from build123d import *

# Parameters (mm, degrees)
SKETCH_2_W            = 36.9
SKETCH_2_H            = 60.6
SKETCH_2_W_2          = 33.7
SKETCH_2_H_2          = 57.4
SKETCH_2_R            = 3.75
SKETCH_2_R_2          = 2.25
SKETCH_2_R_3          = 0.75
EXTRUDE_1_DEPTH       = 1.5
EXTRUDE_2_OUTLINE_R   = 2.154871705
EXTRUDE_2_DEPTH       = 3
EXTRUDE_2_DRAFT       = 28
EXTRUDE_2_2_OUTLINE_R = 2.154871705
EXTRUDE_2_2_DEPTH     = 3
EXTRUDE_2_2_DRAFT     = 28
EXTRUDE_2_3_DEPTH     = 3
EXTRUDE_2_3_DRAFT     = 28
EXTRUDE_2_4_OUTLINE_R = 2.154871705
EXTRUDE_2_4_DEPTH     = 3
EXTRUDE_2_4_DRAFT     = 28
EXTRUDE_START         = 1.5
SKETCH_2_11_W         = 36.9
SKETCH_2_11_H         = 60.6
SKETCH_2_11_W_2       = 33.7
SKETCH_2_11_H_2       = 57.4
EXTRUDE_3_DEPTH       = 4.5
SKETCH_3_W            = 1.6
SKETCH_3_H            = 5.7
SKETCH_3_H_2          = 5.5
EXTRUDE_4_DEPTH       = 4.3
SKETCH_5_W            = 0.8
SKETCH_5_H            = 5.5
SKETCH_5_H_2          = 5.7
EXTRUDE_5_DEPTH       = 1.5
CUT_EXTRUDE_START     = 1.5
SKETCH_2_12_R         = 0.75
CUT_EXTRUDE_1_DEPTH   = 3


# Read off the part's stored shape, not the designer's step: Бобышка-Вытянуть2
with BuildPart() as part:
    # Эскиз2 → Бобышка-Вытянуть1 (new body)
    # profile 1 of 14: a face of its own
    with BuildSketch(Plane(origin=(0, 0, 0), x_dir=(1, 0, 0), z_dir=(0, 1, 0))):
        with Locations((16.65, 28.5)):
            Rectangle(SKETCH_2_W, SKETCH_2_H)
        with Locations((16.65, 28.5)):
            Rectangle(SKETCH_2_W_2, SKETCH_2_H_2, mode=Mode.SUBTRACT)
    # profile 2 of 14: a face of its own
    with BuildSketch(Plane(origin=(0, 0, 0), x_dir=(1, 0, 0), z_dir=(0, 1, 0))):
        with BuildLine():
            Line((-0.2, 57.2), (-0.2, -0.2))
            Line((-0.2, -0.2), (33.5, -0.2))
            Line((33.5, -0.2), (33.5, 10.050490243))
            ThreePointArc((33.5, 10.050490243), (27, 12.6), (33.5, 15.149509757))
            Line((33.5, 15.149509757), (33.5, 57.2))
            Line((33.5, 57.2), (-0.2, 57.2))
        make_face()
        with Locations((5.1, 19.73)):
            Circle(SKETCH_2_R, mode=Mode.SUBTRACT)
        with Locations((5.1, 41.13)):
            Circle(SKETCH_2_R, mode=Mode.SUBTRACT)
        with Locations((23.55, 45)):
            Circle(SKETCH_2_R, mode=Mode.SUBTRACT)
    # profile 3 of 14: a face of its own
    with BuildSketch(Plane(origin=(0, 0, 0), x_dir=(1, 0, 0), z_dir=(0, 1, 0))):
        with Locations((23.55, 45)):
            Circle(SKETCH_2_R)
        with Locations((23.55, 45)):
            Circle(SKETCH_2_R_2, mode=Mode.SUBTRACT)
    # profile 4 of 14: a face of its own
    with BuildSketch(Plane(origin=(0, 0, 0), x_dir=(1, 0, 0), z_dir=(0, 1, 0))):
        with Locations((23.55, 45)):
            Circle(SKETCH_2_R_2)
        with Locations((23.55, 45)):
            Circle(SKETCH_2_R_3, mode=Mode.SUBTRACT)
    # profile 5 of 14: a face of its own
    with BuildSketch(Plane(origin=(0, 0, 0), x_dir=(1, 0, 0), z_dir=(0, 1, 0))):
        with Locations((23.55, 45)):
            Circle(SKETCH_2_R_3)
    # profile 6 of 14: a face of its own
    with BuildSketch(Plane(origin=(0, 0, 0), x_dir=(1, 0, 0), z_dir=(0, 1, 0))):
        with Locations((5.1, 41.13)):
            Circle(SKETCH_2_R)
        with Locations((5.1, 41.13)):
            Circle(SKETCH_2_R_2, mode=Mode.SUBTRACT)
    # profile 7 of 14: a face of its own
    with BuildSketch(Plane(origin=(0, 0, 0), x_dir=(1, 0, 0), z_dir=(0, 1, 0))):
        with Locations((5.1, 41.13)):
            Circle(SKETCH_2_R_2)
        with Locations((5.1, 41.13)):
            Circle(SKETCH_2_R_3, mode=Mode.SUBTRACT)
    # profile 8 of 14: a face of its own
    with BuildSketch(Plane(origin=(0, 0, 0), x_dir=(1, 0, 0), z_dir=(0, 1, 0))):
        with Locations((5.1, 41.13)):
            Circle(SKETCH_2_R_3)
    # profile 9 of 14: a face of its own
    with BuildSketch(Plane(origin=(0, 0, 0), x_dir=(1, 0, 0), z_dir=(0, 1, 0))):
        with Locations((5.1, 19.73)):
            Circle(SKETCH_2_R)
        with Locations((5.1, 19.73)):
            Circle(SKETCH_2_R_2, mode=Mode.SUBTRACT)
    # profile 10 of 14: a face of its own
    with BuildSketch(Plane(origin=(0, 0, 0), x_dir=(1, 0, 0), z_dir=(0, 1, 0))):
        with Locations((5.1, 19.73)):
            Circle(SKETCH_2_R_2)
        with Locations((5.1, 19.73)):
            Circle(SKETCH_2_R_3, mode=Mode.SUBTRACT)
    # profile 11 of 14: a face of its own
    with BuildSketch(Plane(origin=(0, 0, 0), x_dir=(1, 0, 0), z_dir=(0, 1, 0))):
        with Locations((5.1, 19.73)):
            Circle(SKETCH_2_R_3)
    # profile 12 of 14: a face of its own
    with BuildSketch(Plane(origin=(0, 0, 0), x_dir=(1, 0, 0), z_dir=(0, 1, 0))):
        with BuildLine():
            ThreePointArc((33.5, 15.149509757), (27, 12.6), (33.5, 10.050490243))
            Line((33.5, 10.050490243), (33.5, 15.149509757))
        make_face()
        with Locations((30.75, 12.6)):
            Circle(SKETCH_2_R_2, mode=Mode.SUBTRACT)
    # profile 13 of 14: a face of its own
    with BuildSketch(Plane(origin=(0, 0, 0), x_dir=(1, 0, 0), z_dir=(0, 1, 0))):
        with Locations((30.75, 12.6)):
            Circle(SKETCH_2_R_2)
        with Locations((30.75, 12.6)):
            Circle(SKETCH_2_R_3, mode=Mode.SUBTRACT)
    # profile 14 of 14: a face of its own
    with BuildSketch(Plane(origin=(0, 0, 0), x_dir=(1, 0, 0), z_dir=(0, 1, 0))):
        with Locations((30.75, 12.6)):
            Circle(SKETCH_2_R_3)
    extrude(amount=EXTRUDE_1_DEPTH)


with BuildPart() as extrude_2_tool:
    # Бобышка-Вытянуть2 outline → Бобышка-Вытянуть2 (with draft: the straight prism first)
    with BuildSketch(Plane(origin=(0, 4.5, 0), x_dir=(1, 0, 0), z_dir=(0, 1, 0))):
        with Locations((5.1, 41.13)):
            Circle(EXTRUDE_2_OUTLINE_R)
    extrude(amount=-EXTRUDE_2_DEPTH)
    # Бобышка-Вытянуть2: the draft: its side faces are tilted about the plane it starts from
    extrude_2_sides = [extrude_2_tool.faces().sort_by_distance(p)[0] for p in [
        (2.945128295, 3, -41.13),
    ]]
    draft(extrude_2_sides, Plane(origin=(0, 4.5, 0), x_dir=(1, 0, 0), z_dir=(0, 1, 0)), EXTRUDE_2_DRAFT)


with BuildPart() as part_1:
    add(part.part)

    # Бобышка-Вытянуть2: add extrude_2_tool
    add(extrude_2_tool.part)


with BuildPart() as extrude_2_2_tool:
    # Extrude 2 2 outline → Extrude 2 2 (with draft: the straight prism first)
    with BuildSketch(Plane(origin=(0, 4.5, 0), x_dir=(1, 0, 0), z_dir=(0, 1, 0))):
        with Locations((23.55, 45)):
            Circle(EXTRUDE_2_2_OUTLINE_R)
    extrude(amount=-EXTRUDE_2_2_DEPTH)
    # Extrude 2 2: the draft: its side faces are tilted about the plane it starts from
    extrude_2_2_sides = [extrude_2_2_tool.faces().sort_by_distance(p)[0] for p in [
        (21.395128295, 3, -45),
    ]]
    draft(extrude_2_2_sides, Plane(origin=(0, 4.5, 0), x_dir=(1, 0, 0), z_dir=(0, 1, 0)), EXTRUDE_2_2_DRAFT)


with BuildPart() as part_2:
    add(part_1.part)

    # Extrude 2 2: add extrude_2_2_tool
    add(extrude_2_2_tool.part)


with BuildPart() as extrude_2_3_tool:
    # Extrude 2 3 outline → Extrude 2 3 (with draft: the straight prism first)
    with BuildSketch(Plane(origin=(0, 4.5, 0), x_dir=(1, 0, 0), z_dir=(0, 1, 0))):
        with BuildLine():
            ThreePointArc((31.904871705, 14.419270021), (28.595128295, 12.6), (31.904871705, 10.780729979))
            Line((31.904871705, 10.780729979), (31.904871705, 14.419270021))
        make_face()
    extrude(amount=-EXTRUDE_2_3_DEPTH)
    # Extrude 2 3: the draft: its side faces are tilted about the plane it starts from
    extrude_2_3_sides = [extrude_2_3_tool.faces().sort_by_distance(p)[0] for p in [
        (28.595128295, 3, -12.6),
        (31.904871705, 3, -12.6),
    ]]
    draft(extrude_2_3_sides, Plane(origin=(0, 4.5, 0), x_dir=(1, 0, 0), z_dir=(0, 1, 0)), EXTRUDE_2_3_DRAFT)


with BuildPart() as part_3:
    add(part_2.part)

    # Extrude 2 3: add extrude_2_3_tool
    add(extrude_2_3_tool.part)


with BuildPart() as extrude_2_4_tool:
    # Extrude 2 4 outline → Extrude 2 4 (with draft: the straight prism first)
    with BuildSketch(Plane(origin=(0, 4.5, 0), x_dir=(1, 0, 0), z_dir=(0, 1, 0))):
        with Locations((5.1, 19.73)):
            Circle(EXTRUDE_2_4_OUTLINE_R)
    extrude(amount=-EXTRUDE_2_4_DEPTH)
    # Extrude 2 4: the draft: its side faces are tilted about the plane it starts from
    extrude_2_4_sides = [extrude_2_4_tool.faces().sort_by_distance(p)[0] for p in [
        (2.945128295, 3, -19.73),
    ]]
    draft(extrude_2_4_sides, Plane(origin=(0, 4.5, 0), x_dir=(1, 0, 0), z_dir=(0, 1, 0)), EXTRUDE_2_4_DRAFT)


with BuildPart() as part_4:
    add(part_3.part)

    # Extrude 2 4: add extrude_2_4_tool
    add(extrude_2_4_tool.part)

    # Эскиз2<11> → Бобышка-Вытянуть3 (add)
    with BuildSketch(Plane(origin=(0, 0, 0), x_dir=(1, 0, 0), z_dir=(0, 1, 0)).offset(EXTRUDE_START)):
        with Locations((16.65, 28.5)):
            Rectangle(SKETCH_2_11_W, SKETCH_2_11_H)
        with Locations((16.65, 28.5)):
            Rectangle(SKETCH_2_11_W_2, SKETCH_2_11_H_2, mode=Mode.SUBTRACT)
    extrude(amount=EXTRUDE_3_DEPTH)

    # Эскиз3 → Бобышка-Вытянуть4 (add)
    with BuildSketch(Plane(origin=(0, 6, 0), x_dir=(1, 0, 0), z_dir=(0, 1, 0))):
        Polygon((-0.2, 1.3), (-1.8, 1.3), (-1.8, -1.8), (35.1, -1.8), (35.1, 58.8), (-1.8, 58.8), (-1.8, 56.2), (-0.2, 56.2), (-0.2, 57.2), (33.5, 57.2), (33.5, -0.2), (-0.2, -0.2), align=None)
        with Locations((-1, 19.55)):
            Rectangle(SKETCH_3_W, SKETCH_3_H)
        with Locations((-1, 40.95)):
            Rectangle(SKETCH_3_W, SKETCH_3_H_2)
    extrude(amount=EXTRUDE_4_DEPTH)

    # Эскиз5 → Бобышка-Вытянуть5 (add)
    with BuildSketch(Plane(origin=(0, 10.3, 0), x_dir=(1, 0, 0), z_dir=(0, 1, 0))):
        Polygon((-1, -1), (34.3, -1), (34.3, 58), (-1, 58), (-1, 56.2), (-0.2, 56.2), (-0.2, 57.2), (33.5, 57.2), (33.5, -0.2), (-0.2, -0.2), (-0.2, 1.3), (-1, 1.3), align=None)
        with Locations((-0.6, 40.95)):
            Rectangle(SKETCH_5_W, SKETCH_5_H)
        with Locations((-0.6, 19.55)):
            Rectangle(SKETCH_5_W, SKETCH_5_H_2)
    extrude(amount=EXTRUDE_5_DEPTH)

    # Эскиз2<12> → Вырез-Вытянуть1 (cut)
    with BuildSketch(Plane(origin=(0, 0, 0), x_dir=(1, 0, 0), z_dir=(0, 1, 0)).offset(CUT_EXTRUDE_START)):
        with Locations(Location((23.55, 45, 0), (0, 0, 270))):
            Circle(SKETCH_2_12_R)
        with Locations(Location((5.1, 41.13, 0), (0, 0, 270))):
            Circle(SKETCH_2_12_R)
        with Locations(Location((5.1, 19.73, 0), (0, 0, 270))):
            Circle(SKETCH_2_12_R)
        with Locations(Location((30.75, 12.6, 0), (0, 0, 270))):
            Circle(SKETCH_2_12_R)
    extrude(amount=CUT_EXTRUDE_1_DEPTH, mode=Mode.SUBTRACT)


solid = part_4.part
The model under review builds one solid part; all positions refer to its coordinate system, in mm. A direction names the side the tool comes from. Coordinates: 2 decimals unless noted, no trailing zeros. Write each loop counter-clockwise with the first axis right and the second up, starting at its lowest first coordinate (ties: lowest second). Pieces come first, ordered by that corner, then holes. Notation, with made-up numbers: (47.25, 35.25) -> (96.25, 35.25) arc R12 cw to (96.25, 46.25) -> close; hole circle Ø5 at (78, 53.25). An arc over 180 degrees is marked (long way). Answer in a Markdown table with one row per item.
1. Clearance check with flat-ended pins moving along their axes: pin 1 Ø1.6 at (x, z) = (30.5, -12.5) entering from +Y; pin 2 Ø1.8 at (x, z) = (-1.5, -29) entering from +Y; pin 3 Ø12 at (x, z) = (11, -48) entering from +Y. State where each tip first meets the part, or that it passes through.
Answers below:
| item | result |
|---|---|
| pin 1 | stops at y = 4.5 |
| pin 2 | stops at y = 6 |
| pin 3 | stops at y = 2.81 |
2. We need section C-C, the plane x = 13.5. State the section outline as (y, z) points.
Answers below:
| item | result |
|---|---|
| outline | (0, -58.8) -> (10.3, -58.8) -> (10.3, -58) -> (11.8, -58) -> (11.8, -57.2) -> (1.5, -57.2) -> (1.5, 0.2) -> (11.8, 0.2) -> (11.8, 1) -> (10.3, 1) -> (10.3, 1.8) -> (0, 1.8) -> close |
3. We need section B-B, the plane z = -12.6. State the section outline as (x, y) points, and give its area (3 significant figures).
Answers below:
| item | result |
|---|---|
| outline | (-1.8, 0) -> (35.1, 0) -> (35.1, 10.3) -> (34.3, 10.3) -> (34.3, 11.8) -> (33.5, 11.8) -> (33.5, 1.5) -> (31.9, 4.5) -> (31.5, 4.5) -> (31.5, 1.5) -> (30, 1.5) -> (30, 4.5) -> (28.6, 4.5) -> (27, 1.5) -> (-0.2, 1.5) -> (-0.2, 6) -> (-1.8, 6) -> close |
| area | 88.0 mm^2 |
4. For faces 4 (the flat face through (-1, 6, -50)), 5 (the flat face through (17, 7, 0.2)), 6 (the flat face through (35.1, 5, -28)), list the 3-axis set-ups (+Z, -Z, +X, -X, +Y, -Y) from which the entire face can be reached by the end or side of a thin tool; tool diameter is ignored.
Answers below:
| item | result |
|---|---|
| face 4 | -X, +Y |
| face 5 | +Y |
| face 6 | +Z, -Z, +X, +Y, -Y |
5. We need section A-A, the plane y = 8. State the section outline as (x, z) points.
Answers below:
| item | result |
|---|---|
| outline | (-1.8, -58.8) -> (35.1, -58.8) -> (35.1, 1.8) -> (-1.8, 1.8) -> (-1.8, -1.3) -> (-0.2, -1.3) -> (-0.2, 0.2) -> (33.5, 0.2) -> (33.5, -57.2) -> (-0.2, -57.2) -> (-0.2, -56.2) -> (-1.8, -56.2) -> close; (-1.8, -43.7) -> (-0.2, -43.7) -> (-0.2, -38.2) -> (-1.8, -38.2) -> close; (-1.8, -22.4) -> (-0.2, -22.4) -> (-0.2, -16.7) -> (-1.8, -16.7) -> close |
6. Draft analysis for pull direction Z (two halves, no side actions). For faces 1 (the flat face through (5, 1.5, -41)), 2 (the flat face through (17, 5, -58.8)), 3 (the flat face through (-1.8, 4, -29)), state which applies: +Z half, -Z half, draft (parallel to the pull), parting line (faces both ways), or undercut.
Answers below:
| item | result |
|---|---|
| face 1 | undercut |
| face 2 | -Z half |
| face 3 | draft |
7. Wall thickness on probe 1 along Z at (x, y) = (25.5, 11); probe 2 along X at (y, z) = (3.5, -45); probe 3 along Z at (x, y) = (22, 9.75): over which ranges is each line inside the solid? List them lowest first. Write a range as [from, to].
Answers below:
| item | result |
|---|---|
| probe 1 | z = [-58, -57.2], [0.2, 1] |
| probe 2 | x = [-1.8, -0.2], [20.86, 22.8], [24.3, 26.24], [33.5, 35.1] |
| probe 3 | z = [-58.8, -57.2], [0.2, 1.8] |
8. We need section D-D, the plane z = -4.5. State the section outline as (x, y) points.
Answers below:
| item | result |
|---|---|
| outline | (-1.8, 0) -> (35.1, 0) -> (35.1, 10.3) -> (34.3, 10.3) -> (34.3, 11.8) -> (33.5, 11.8) -> (33.5, 1.5) -> (-0.2, 1.5) -> (-0.2, 6) -> (-1.8, 6) -> close |
